from build123d import *

# Parameters (mm, degrees)
BOSS_EXTRUDE1_DEPTH = 30
SKETCH2_R           = 4
CUT_EXTRUDE1_DEPTH  = 31
SKETCH3_R           = 1.5
CUT_EXTRUDE2_DEPTH  = 19.5


with BuildPart() as part:
    # Sketch1 → Boss-Extrude1 (new body)
    with BuildSketch(Plane.XY):
        Polygon((0, 0), (6.25, 0), (7.25, -1), (17.25, -1), (17.25, 5.5), (16.25, 6.5), (16.25, 16.5), (15.25, 17.5), (10.25, 17.5), (5, 21.332427429), (-5, 21.332427429), (-10.25, 17.5), (-15.25, 17.5), (-16.25, 16.5), (-16.25, 6.5), (-17.25, 5.5), (-17.25, -1), (-7.25, -1), (-6.25, 0), align=None)
    extrude(amount=BOSS_EXTRUDE1_DEPTH)

    # Sketch2 → Cut-Extrude1 (cut, through all)
    with BuildSketch(Plane.XY.offset(30)):
        with Locations((0, 9.332427429)):
            Circle(SKETCH2_R)
    extrude(amount=-CUT_EXTRUDE1_DEPTH, mode=Mode.SUBTRACT)

    # Sketch3 → Cut-Extrude2 (cut, through all)
    with BuildSketch(Plane(origin=(0, 17.5, 0), x_dir=(1, 0, 0), z_dir=(0, 1, 0))):
        with Locations((12.25, -6)):
            Circle(SKETCH3_R)
        with Locations((12.25, -24)):
            Circle(SKETCH3_R)
    cut_extrude2 = extrude(amount=-CUT_EXTRUDE2_DEPTH, mode=Mode.SUBTRACT)

    # Mirror1: Cut-Extrude2 across plane
    add(cut_extrude2.mirror(Plane(origin=(0, 0, 0), x_dir=(0, 0, 1), z_dir=(1, 0, 0))), mode=Mode.SUBTRACT)


solid = part.part
Work out the finished part from the listing and answer in its coordinate system (mm). A direction names the side the tool comes from. Round coordinates to 2 decimals unless told otherwise and drop trailing zeros. Order: outer loops, then holes, each group sorted by start corner. A loop starts at its lowest first (then second) coordinate and runs counter-clockwise, first axis right, second up. Notation, with made-up numbers: M 77.25,51.25 L 101.25,51.25 A24 cw 101.25,90.25 Z; hole C 49,-35 d5. An arc over 180 degrees is marked long. Put each result on its own line as item: value. Start each with the question number.
Q1. Section C-C, the plane x = 0 is taken. Write down the section's boundary in (y, z), and give its area (3 significant figures).
Q2. For a pull along X with two mould halves and no side action, classify faces 1 (the flat face through (-16.25, 12, 15)), 2 (the flat face through (0, 0, 15)), 3 (the flat face through (15.76, 16.99, 14.79)) as pulls with the +X half, pulls with the -X half, needs draft (parallel to the pull), parting line crosses it, or undercut.
Q3. Section B-B, the plane y = 2.5 is taken. Write down the section's boundary in (x, z).
Q4. Flat-ended cylindrical pins translate along their axes: pin 1 (11 mm diameter, centred on y = 10.5, z = 10, fed in from +X); pin 2 (1 mm diameter, centred on x = 6, z = 11.5, fed in from -Y); pin 3 (4 mm diameter, centred on x = -12.5, z = 17.5, fed in from +Y); pin 4 (4 mm diameter, centred on x = 1.5, z = 11.5, fed in from -Y). Find the tip coordinate at first contact, or state that the pin passes through.
Q5. Section A-A, the plane x = -12.25 is taken. Write down the section's boundary in (y, z).
Q6. Straight lines are drawn through the part: L1, parallel to Z at x = 12.25, y = 13.75; L2, parallel to Y at x = 0, z = 14.5; L3, parallel to X at y = 7.75, z = 6. For each, find the intervals that lie inside material, in ascending order. Write a range as [from, to].
Q7. Section D-D, the plane z = 24 is taken. Write down the section's boundary in (x, y), and give its area (3 significant figures).
Q8. A tool of negligible diameter and unlimited length cuts with its end or side. For faces 4 (the flat face through (-13, 17.5, 15)), 5 (the cylindrical face through (-10.75, 8.38, 5.93)), 6 (the flat face through (16.25, 11, 15)), from which of +Z, -Z, +X, -X, +Y, -Y can it reach the whole face along a straight path? Write none if from no direction.
Findings below:
1. outline: M 0,0 L 5.33,0 L 5.33,30 L 0,30 Z; M 13.33,0 L 21.33,0 L 21.33,30 L 13.33,30 Z
1. area: 400 mm^2
2. face 1: pulls with the -X half
2. face 2: undercut
2. face 3: pulls with the +X half
3. outline: M -17.25,0 L 17.25,0 L 17.25,30 L -17.25,30 Z; hole C -12.25,6 d3; hole C -12.25,24 d3; hole C 12.25,6 d3; hole C 12.25,24 d3
4. pin 1: stops at x = 17.25
4. pin 2: stops at y = -0.25
4. pin 3: stops at y = 17.5
4. pin 4: stops at y = 0
5. outline: M -1,0 L 17.5,0 L 17.5,4.5 L -1,4.5 Z; M -1,7.5 L 17.5,7.5 L 17.5,22.5 L -1,22.5 Z; M -1,25.5 L 17.5,25.5 L 17.5,30 L -1,30 Z
6. L1: z = [0, 4.5], [7.5, 22.5], [25.5, 30]
6. L2: y = [0, 5.33], [13.33, 21.33]
6. L3: x = [-16.25, -13.75], [-10.75, -3.67], [3.67, 10.75], [13.75, 16.25]
7. outline: M -17.25,-1 L -13.75,-1 L -13.75,17.5 L -15.25,17.5 L -16.25,16.5 L -16.25,6.5 L -17.25,5.5 Z; M -10.75,-1 L -7.25,-1 L -6.25,0 L 6.25,0 L 7.25,-1 L 10.75,-1 L 10.75,17.5 L 10.25,17.5 L 5,21.33 L -5,21.33 L -10.25,17.5 L -10.75,17.5 Z; M 13.75,-1 L 17.25,-1 L 17.25,5.5 L 16.25,6.5 L 16.25,16.5 L 15.25,17.5 L 13.75,17.5 Z; hole C 0,9.33 d8
7. area: 498 mm^2
8. face 4: +Z, -Z, -X, +Y
8. face 5: +Y, -Y
8. face 6: +Z, -Z, +X, +Y
